from build123d import *

# Parameters (mm, degrees)
SKETCH2_R           = 6
BOSS_EXTRUDE1_DEPTH = 4.7625
FILLET1_R           = 5


with BuildPart() as part:
    # Sketch2 → Boss-Extrude1 (new body)
    with BuildSketch(Plane(origin=(0, 0, 0), x_dir=(1, 0, 0), z_dir=(0, 1, 0))):
        with BuildLine():
            Line((-122.387926706, -10), (-0.763550737, -15.856626857))
            ThreePointArc((-0.763550737, -15.856626857), (15.875, -1.57e-07), (-0.763550423, 15.856626872))
            Line((-0.763550423, 15.856626872), (-122.387926706, 10))
            Line((-122.387926706, 10), (-122.387926706, -10))
        make_face()
        with Locations((-112.387926706, 0)):
            Circle(SKETCH2_R, mode=Mode.SUBTRACT)
    extrude(amount=BOSS_EXTRUDE1_DEPTH)

    # Fillet1
    fillet1_edges = [part.edges().sort_by_distance(p)[0] for p in [
        (-122.387926706, 2.38125, 10),
        (-122.387926706, 2.38125, -10),
    ]]
    fillet(fillet1_edges, radius=FILLET1_R)


solid = part.part
Here's how the part is built. I have some questions about the finished solid (model axes, mm). Give positions to 0.01 mm unless a question says otherwise; leave off trailing zeros. Loops run counter-clockwise (first coordinate to the right, second up) from the corner with the lowest first, then second, coordinate; pieces in that order, holes last. Notation, with made-up numbers: (18.5, 7) -> (64.5, 7) arc R29 ccw to (64.5, 40) -> close; hole circle Ø1 at (85, -1.5). An arc over 180 degrees is marked (long way). One line per item, written item: value.
Q1. If I drill on line 1 along Z through (x, y) = (-115.5, 3.7); line 2 along Z through (x, y) = (-22, 4.05); line 3 along Z through (x, y) = (-15, 3.1), over which ranges is the centre line in solid material (lowest first)?
Answers follow:
line 1: -10.33 to -5.13, 5.13 to 10.33
line 2: -14.83 to 14.83
line 3: -15.17 to 15.17
Q2. I'm going to push flat-ended pins straight in: pin 1 Ø1 at (x, y) = (-101.5, 4) entering from +Z; pin 2 Ø1 at (y, z) = (3.5, -12) entering from +X; pin 3 Ø9.5 at (x, z) = (-112.39, 0) entering from +Y. Where does each tip first touch, or does it pass through?
Answers follow:
pin 1: z = 11.03
pin 2: x = 10.94
pin 3: through
Q3. Suppose I cut it at A-A on z = 0. Please give me the cut outline in (x, y) (1 decimal).
Answers follow:
outline: (-122.4, 0) -> (-118.4, 0) -> (-118.4, 4.8) -> (-122.4, 4.8) -> close; (-106.4, 0) -> (15.9, 0) -> (15.9, 4.8) -> (-106.4, 4.8) -> close
Q4. Suppose I cut it at D-D on z = 13. Please give me the cut outline in (x, y), then the cut area to 3 significant figures.
Answers follow:
outline: (-60.09, 0) -> (9.11, 0) -> (9.11, 4.76) -> (-60.09, 4.76) -> close
area: 330 mm^2
Q5. Suppose I cut it at C-C on x = -46. Please give me the cut outline in (y, z), then the cut area to 3 significant figures.
Answers follow:
outline: (0, -13.68) -> (4.76, -13.68) -> (4.76, 13.68) -> (0, 13.68) -> close
area: 130 mm^2
Q6. Suppose I cut it at B-B on y = 3.8. Please give me the cut outline in (x, z) (3 decimals).
Answers follow:
outline: (-122.388, -5.235) arc R5 ccw to (-117.628, -10.229) -> (-0.764, -15.857) arc R15.875 ccw (long way) to (-0.764, 15.857) -> (-117.628, 10.229) arc R5 ccw to (-122.388, 5.235) -> close; hole circle Ø12 at (-112.388, 0)
Q7. We'd pull the mould along X, two halves only. Please class faces 1 (the face through (-58.378, 2.348, -13.082)), 2 (the face through (-118.382, 2.348, -0.264)), 3 (the face through (-39, 4.762, 0)): pulls with the +X half, pulls with the -X half, needs draft (parallel to the pull), parting line crosses it, or undercut.
Answers follow:
face 1: pulls with the -X half
face 2: undercut
face 3: needs draft
